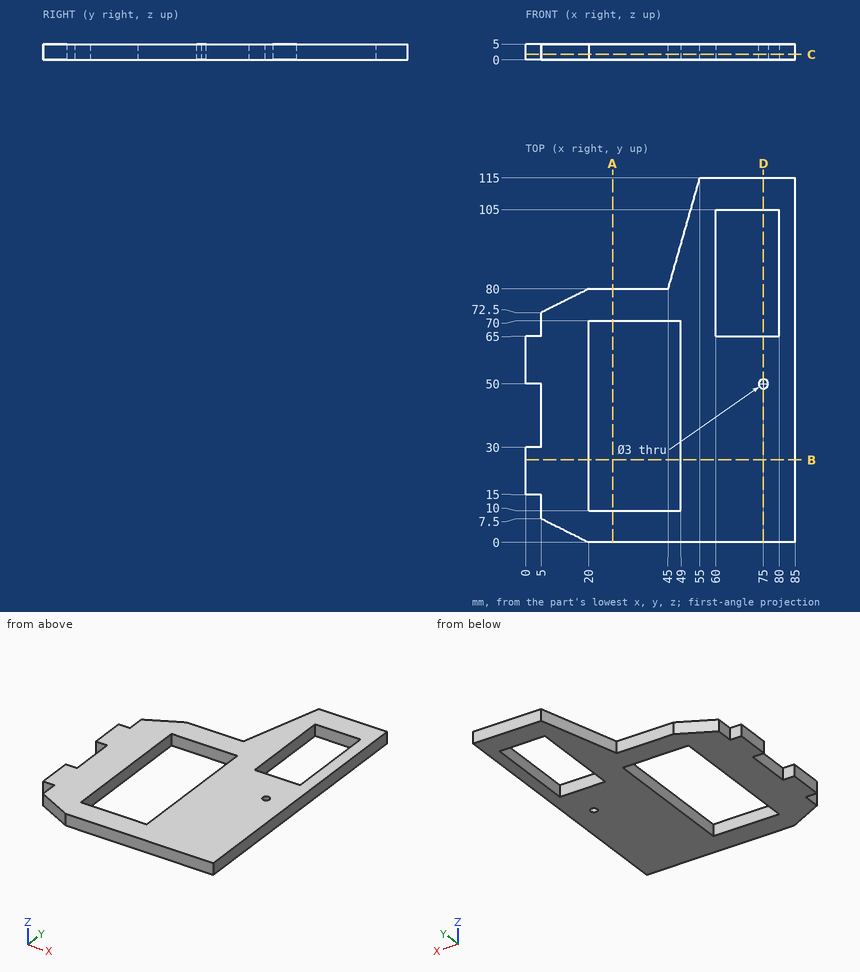
For this review, use the dimensioned drawing (mm, ordinates from the lowest corner) and the shaded views. Coordinates: 2 decimals unless noted, no trailing zeros. Loops run counter-clockwise (first coordinate to the right, second up) from the corner with the lowest first, then second, coordinate; pieces in that order, holes last. Notation, with made-up numbers: (-30, 9) -> (-17, 9) arc R36 cw to (-17, 46) -> close; hole circle Ø3 at (47.5, 61.25). An arc over 180 degrees is marked (long way). Return JSON: item names as keys, results as strings. Group by question number.
(1) For pin 1 Ø1.5 at (x, z) = (67, 2.5) entering from -Y; pin 2 Ø1.5 at (y, z) = (68.5, 2) entering from -X; pin 3 Ø1.5 at (x, z) = (1.5, 3.5) entering from +Y; pin 4 Ø2.5 at (x, z) = (39.5, 3.5) entering from +Y, all flat-tipped, find the tip position at first contact; note any pin that passes through.
(2) To check wall thickness, follow L1, parallel to Y at x = 75, z = 2.4; L2, parallel to X at y = 15.5, z = 2.45; L3, parallel to X at y = 35.5, z = 1.55. State the ranges of each line that lie inside material, in increasing order.
(3) Consider section D-D, the plane x = 75. Give the boundary of the cut face in (y, z), plus the area to 3 significant figures.
(4) Consider section C-C, the plane z = 1.7. Give the boundary of the cut face in (x, y), plus the area to 3 significant figures.
(5) Consider section B-B, the plane y = 26. Give the boundary of the cut face in (x, z), plus the area to 3 significant figures.
(6) Consider section A-A, the plane x = 27.5. Give the boundary of the cut face in (y, z).
Results below:
{
 "1": {"pin 1": "stops at y = 0", "pin 2": "stops at x = 5", "pin 3": "stops at y = 65", "pin 4": "stops at y = 80"},
 "2": {"L1": "y = 0 to 48.5, 51.5 to 65, 105 to 115", "L2": "x = 0 to 20, 49 to 85", "L3": "x = 5 to 20, 49 to 85"},
 "3": {"outline": "(0, 0) -> (48.5, 0) -> (48.5, 5) -> (0, 5) -> close; (51.5, 0) -> (65, 0) -> (65, 5) -> (51.5, 5) -> close; (105, 0) -> (115, 0) -> (115, 5) -> (105, 5) -> close", "area": "360 mm2"},
 "4": {"outline": "(0, 15) -> (5, 15) -> (5, 7.5) -> (20, 0) -> (85, 0) -> (85, 115) -> (55, 115) -> (45, 80) -> (20, 80) -> (5, 72.5) -> (5, 65) -> (0, 65) -> (0, 50) -> (5, 50) -> (5, 30) -> (0, 30) -> close; hole (20, 10) -> (49, 10) -> (49, 70) -> (20, 70) -> close; hole (60, 65) -> (80, 65) -> (80, 105) -> (60, 105) -> close; hole circle Ø3 at (75, 50)", "area": "5,120 mm2"},
 "5": {"outline": "(0, 0) -> (20, 0) -> (20, 5) -> (0, 5) -> close; (49, 0) -> (85, 0) -> (85, 5) -> (49, 5) -> close", "area": "280 mm2"},
 "6": {"outline": "(0, 0) -> (10, 0) -> (10, 5) -> (0, 5) -> close; (70, 0) -> (80, 0) -> (80, 5) -> (70, 5) -> close"}
}
